from build123d import *

# Parameters (mm, degrees)
F1_DEPTH    = 4
F2_R        = 8
F3_DEPTH    = 25
F4_T1_DEPTH = 50.4194138592
F4_T3_DEPTH = 170.6048746571


# Not quite as in the source:
# - a fillet or chamfer that OpenCascade refuses, or shapes differently, is made with other operations: its cross-section is extruded or revolved along the edge and cut away or added


with BuildPart() as f1:
    # F0 (on Top) → F1 (new body)
    with BuildSketch(Plane.XY):
        Polygon((65, 0), (65, 25), (0, 25), (-65, 0), (-65, -25), (0, -25), align=None)
    extrude(amount=F1_DEPTH)

    # F2 (on face) → F3 (cut)
    with BuildSketch(Plane.XY.offset(4)):
        Circle(F2_R)
    extrude(amount=-F3_DEPTH, mode=Mode.SUBTRACT)

    # F4: fillet of radius 50 on 4 edges, made by hand

    # F4_s2 → F4_t1 (cut)
    with BuildSketch(Plane.XY.offset(-23.2097069296)):
        with BuildLine():
            ThreePointArc((8.6650711936, -21.6672803102), (-0.1560137847, -24.1597600457), (-9.2838827718, -25))
            Line((-9.2838827718, -25), (0, -25))
            Line((0, -25), (8.6650711936, -21.6672803102))
        make_face()
        with BuildLine():
            ThreePointArc((9.2838827718, 25), (0.1560137847, 24.1597600457), (-8.6650711936, 21.6672803102))
            Line((-8.6650711936, 21.6672803102), (0, 25))
            Line((0, 25), (9.2838827718, 25))
        make_face()
    extrude(amount=F4_T1_DEPTH, mode=Mode.SUBTRACT)

    # F4_s4 → F4_t3 (cut)
    with BuildSketch(Plane.XY.offset(-83.3024373285)):
        with BuildLine():
            ThreePointArc((-33.9000144534, 11.9615329026), (-54.209630263, -2.5144156742), (-65, -25))
            Line((-65, -25), (-65, 0))
            Line((-65, 0), (-33.9000144534, 11.9615329026))
        make_face()
        with BuildLine():
            ThreePointArc((65, 25), (54.209630263, 2.5144156742), (33.9000144534, -11.9615329026))
            Line((33.9000144534, -11.9615329026), (65, 0))
            Line((65, 0), (65, 25))
        make_face()
    extrude(amount=F4_T3_DEPTH, mode=Mode.SUBTRACT)


solid = f1.part
Geometry: final body of the model. Coordinates: model frame, mm. Coordinates: 2 decimals unless noted, no trailing zeros. Order: outer loops, then holes, each group sorted by start corner. A loop starts at its lowest first (then second) coordinate and runs counter-clockwise, first axis right, second up.
(1) Draft query along X for faces 1 (the face through (-1.73, -7.81, 2.03)), 2 (the face through (54.44, 2.79, 1.97)), 3 (the face through (-1, -11, 4)), 4 (the face through (0.282, 24.183, 1.972)). Return one class per face: pulls with the +X half, pulls with the -X half, needs draft (parallel to the pull), parting line crosses it, or undercut.
(2) Section query A-A (z = 1.8). Return the cut outline in (x, y).
(3) Material intervals for probe 1 along Y at (x, z) = (0, 1.8); probe 2 along X at (y, z) = (5, 2.7) (3 decimals); probe 3 along X at (y, z) = (4.5, 2.2), sorted ascending.
(4) First-contact query: pin 1 (1 mm diameter, centred on x = 6, z = 2.5, fed in from -Y); pin 2 (1.5 mm diameter, centred on y = -14, z = 3.5, fed in from -X); pin 3 (13 mm diameter, centred on x = 0, y = 0, fed in from +Z). Flat tips, straight axial feed; report the tip coordinate or a pass-through.
(5) Section query B-B (x = 0). Return the cut outline in (y, z), plus the area to 3 significant figures.
(6) Section query C-C (y = 0). Return the cut outline in (x, z).
(7) Section query D-D (x = -54.5). Return the cut outline in (y, z).
Solution:
1. face 1: undercut
1. face 2: pulls with the +X half
1. face 3: needs draft
1. face 4: pulls with the -X half
2. outline: (-65, -25) - (-9.28, -25) arc R50 ccw to (8.67, -21.67) - (33.9, -11.96) arc R50 ccw to (65, 25) - (9.28, 25) arc R50 ccw to (-8.67, 21.67) - (-33.9, 11.96) arc R50 ccw to start; hole circle Ø16 at (0, 0)
3. probe 1: y = -24.13 to -8, 8 to 24.13
3. probe 2: x = -46.339 to -6.245, 6.245 to 56.17
3. probe 3: x = -46.98 to -6.61, 6.61 to 55.8
4. pin 1: stops at y = -22.76
4. pin 2: stops at x = -61.8
4. pin 3: passes through
5. outline: (-24.13, 0) - (-8, 0) - (-8, 4) - (-24.13, 4) - close; (8, 0) - (24.13, 0) - (24.13, 4) - (8, 4) - close
5. area: 129 mm2
6. outline: (-51.94, 0) - (-8, 0) - (-8, 4) - (-51.94, 4) - close; (8, 0) - (51.94, 0) - (51.94, 4) - (8, 4) - close
7. outline: (-25, 0) - (-2.86, 0) - (-2.86, 4) - (-25, 4) - close
